Read the model definition and answer for the solid it produces. Units are mm, in the model's axes. A direction names the side the tool comes from. Round coordinates to 2 decimals unless told otherwise and drop trailing zeros. Loops run counter-clockwise (first coordinate to the right, second up) from the corner with the lowest first, then second, coordinate; pieces in that order, holes last. Notation, with made-up numbers: M 85,66.5 L 107,66.5 A20 cw 107,74.5 Z; hole C -1.75,66 d9. An arc over 180 degrees is marked long. Answer as CSV lines item,"result".
```python
from build123d import *

# Parameters (mm, degrees)
SKETCH1_W           = 5
SKETCH1_H           = 100
BOSS_EXTRUDE1_DEPTH = 2
SKETCH2_W           = 5
SKETCH2_H           = 2
CUT_EXTRUDE1_DEPTH  = 50
SKETCH3_W           = 5
SKETCH3_H           = 2
CUT_EXTRUDE2_DEPTH  = 20


with BuildPart() as part:
    # Sketch1 → Boss-Extrude1 (new body)
    with BuildSketch(Plane.XY):
        with Locations((5.5, -50)):
            Rectangle(SKETCH1_W, SKETCH1_H)
        with Locations((15.5, -50)):
            Rectangle(SKETCH1_W, SKETCH1_H)
        Polygon((24, 0), (0, 7), (0, 0), align=None)
        Polygon((8.6, 9.7), (18.2, 6.9), (16.8, 2.1), (7.2, 4.9), align=None)
    extrude(amount=BOSS_EXTRUDE1_DEPTH)

    # Sketch2 → Cut-Extrude1 (cut)
    with BuildSketch(Plane.XZ.offset(100)):
        with Locations((5.5, 1)):
            Rectangle(SKETCH2_W, SKETCH2_H)
        with Locations((15.5, 1)):
            Rectangle(SKETCH2_W, SKETCH2_H)
    extrude(amount=-CUT_EXTRUDE1_DEPTH, mode=Mode.SUBTRACT)

    # Sketch3 → Cut-Extrude2 (cut)
    with BuildSketch(Plane(origin=(0, -50, 0), x_dir=(-1, 0, 0), z_dir=(0, -1, 0))):
        with Locations((-5.5, -1)):
            Rectangle(SKETCH3_W, SKETCH3_H)
        with Locations((-15.5, -1)):
            Rectangle(SKETCH3_W, SKETCH3_H)
    extrude(amount=-CUT_EXTRUDE2_DEPTH, mode=Mode.SUBTRACT)


solid = part.part
```
1) A tool of negligible diameter and unlimited length cuts with its end or side. For faces 4 (the flat face through (10, 0, 1)), 5 (the flat face through (3, -15, 1)), 6 (the flat face through (20.45, 1.035, 0.986)), from which of +Z, -Z, +X, -X, +Y, -Y can it reach the whole face along a straight path? Write none if from no direction.
Evaluation:
face 4,"+Z, -Z, -Y"
face 5,"+Z, -Z, -X, -Y"
face 6,"+Z, -Z, +X"
2) Find section A-A, the plane y = -20. Give the vertices of the cut face in (x, z), then the cut area to 3 significant figures.
Evaluation:
outline,"M 3,0 L 8,0 L 8,2 L 3,2 Z; M 13,0 L 18,0 L 18,2 L 13,2 Z"
area,"20.0 mm^2"
3) Find section D-D, the plane y = 1.5. Give the vertices of the cut face in (x, z), then the cut area to 3 significant figures.
Evaluation:
outline,"M 0,0 L 18.86,0 L 18.86,2 L 0,2 Z"
area,"37.7 mm^2"
4) Each of these flat-tipped pins is pushed along its axis until it touches: P1, Ø1, axis at y = -9, z = 1, coming from the -X side; P2, Ø0.6, axis at x = 2, z = 0.5, coming from the -Y side. Where does it stop, or does it pass through?
Evaluation:
P1,"stops at x = 3"
P2,"stops at y = 0"
5) Straight lines are drawn through the part: line 1 (X direction, y = -21, z = 0.9); line 2 (Y direction, x = 4, z = 1.4); line 3 (Y direction, x = 13.5, z = 0.7). For each, find the intervals that lie inside material, in ascending order.
Evaluation:
line 1,"x = 3 to 8, 13 to 18"
line 2,"y = -30 to 5.83"
line 3,"y = -30 to 8.27"
6) Determine the mould class of faces 1 (the flat face through (6, -30, 1)), 2 (the flat face through (13, -15, 1)), 3 (the flat face through (17.5, 4.5, 1)) for opening direction Y: released by +Y, released by -Y, zero draft, split by the parting line, or undercut.
Evaluation:
face 1,"released by -Y"
face 2,"zero draft"
face 3,"undercut"
7) Find section C-C, the plane x = 15.5. Give the vertices of the cut face in (y, z), then the cut area to 3 significant figures.
Evaluation:
outline,"M -30,0 L 7.69,0 L 7.69,2 L -30,2 Z"
area,"75.4 mm^2"
8) Find section B-B, the plane z = 0.55. Give the vertices of the cut face in (x, y), then the cut area to 3 significant figures.
Evaluation:
outline,"M 0,0 L 3,0 L 3,-30 L 8,-30 L 8,0 L 13,0 L 13,-30 L 18,-30 L 18,0 L 24,0 L 16.8,2.1 L 18.2,6.9 L 8.6,9.7 L 7.2,4.9 L 0,7 Z"
area,"434 mm^2"
